Work out the finished part from the listing and answer in its coordinate system (mm). A direction names the side the tool comes from. Round coordinates to 2 decimals unless told otherwise and drop trailing zeros. Order: outer loops, then holes, each group sorted by start corner. A loop starts at its lowest first (then second) coordinate and runs counter-clockwise, first axis right, second up. Notation, with made-up numbers: (45, 32.5) - (96, 32.5) arc R24 ccw to (96, 54.5) - close; hole circle Ø3 at (79.5, 18.25). An arc over 180 degrees is marked (long way). Answer in a Markdown table with one row per item.
from build123d import *

# Parameters (mm, degrees)
SKETCH1_R           = 4.1
SKETCH1_R_2         = 4
SKETCH1_R_3         = 2.6
BOSS_EXTRUDE1_DEPTH = 10
CUT_EXTRUDE1_START  = -4
CUT_EXTRUDE1_DEPTH  = 4
FILLET1_R           = 2
BOSS_EXTRUDE2_START = -20
SKETCH3_R           = 4
BOSS_EXTRUDE2_DEPTH = 20
FILLET2_R           = 1
CUT_EXTRUDE2_REACH  = 75.469


with BuildPart() as part:
    # Sketch1 → Boss-Extrude1 (new body)
    with BuildSketch(Plane(origin=(0, 0, 0), x_dir=(1, 0, 0), z_dir=(0, 1, 0))):
        with BuildLine():
            Line((11.273947383, 72.313413723), (4.792068361, 72.313413723))
            Line((4.792068361, 72.313413723), (-53.726052617, 72.313413723))
            ThreePointArc((-53.726052617, 72.313413723), (-57.261586523, 70.848947629), (-58.726052617, 67.313413723))
            Line((-58.726052617, 67.313413723), (-58.726052617, 34.313413723))
            ThreePointArc((-58.726052617, 34.313413723), (-57.261586523, 30.777879817), (-53.726052617, 29.313413723))
            Line((-53.726052617, 29.313413723), (-5.726052617, 29.313413723))
            ThreePointArc((-5.726052617, 29.313413723), (1.345015195, 26.384481534), (4.273947383, 19.313413723))
            Line((4.273947383, 19.313413723), (4.273947383, 17.313413723))
            ThreePointArc((4.273947383, 17.313413723), (5.738413477, 13.777879817), (9.273947383, 12.313413723))
            Line((9.273947383, 12.313413723), (36.273947383, 12.313413723))
            ThreePointArc((36.273947383, 12.313413723), (39.809481289, 13.777879817), (41.273947383, 17.313413723))
            Line((41.273947383, 17.313413723), (41.273947383, 42.313413723))
            ThreePointArc((41.273947383, 42.313413723), (32.487150819, 63.526617158), (11.273947383, 72.313413723))
        make_face()
        with Locations(Location((33.273947383, 20.313413723, 0), (0, 0, 270))):
            Circle(SKETCH1_R, mode=Mode.SUBTRACT)
        with Locations(Location((12.273947383, 20.313413723, 0), (0, 0, 270))):
            Circle(SKETCH1_R_2, mode=Mode.SUBTRACT)
        with Locations(Location((-50.726052617, 64.313413723, 0), (0, 0, 270))):
            Circle(SKETCH1_R_3, mode=Mode.SUBTRACT)
        with Locations(Location((-50.726052617, 37.313413723, 0), (0, 0, 270))):
            Circle(SKETCH1_R_3, mode=Mode.SUBTRACT)
        with BuildLine():
            Line((34.171420048, 34.313413723), (26.134777641, 34.313413723))
            ThreePointArc((26.134777641, 34.313413723), (25.561526201, 34.49403421), (25.19535667, 34.97064815))
            Line((25.19535667, 34.97064815), (14.615821544, 63.966084002))
            ThreePointArc((14.615821544, 63.966084002), (14.998488248, 65.980552022), (16.952543045, 66.601989919))
            ThreePointArc((16.952543045, 66.601989919), (32.892900514, 54.755368869), (35.127730175, 35.021059585))
            ThreePointArc((35.127730175, 35.021059585), (34.766250218, 34.509562325), (34.171420048, 34.313413723))
        make_face(mode=Mode.SUBTRACT)
        with BuildLine():
            Line((-42.557674575, 35.313413723), (-42.557674575, 60.452375226))
            ThreePointArc((-42.557674575, 60.452375226), (-41.891342574, 61.395065879), (-40.780343242, 61.081466633))
            Line((-40.780343242, 61.081466633), (-20.435473581, 35.94250513))
            ThreePointArc((-20.435473581, 35.94250513), (-20.310283056, 34.882769674), (-21.212804914, 34.313413723))
            Line((-21.212804914, 34.313413723), (-41.557674575, 34.313413723))
            ThreePointArc((-41.557674575, 34.313413723), (-42.264781356, 34.606306941), (-42.557674575, 35.313413723))
        make_face(mode=Mode.SUBTRACT)
        with BuildLine():
            Line((-37.245793747, 67.251595954), (5.443945576, 67.251595954))
            ThreePointArc((5.443945576, 67.251595954), (6.346467434, 66.682240002), (6.221276909, 65.622504547))
            Line((6.221276909, 65.622504547), (-15.123592752, 39.247901728))
            ThreePointArc((-15.123592752, 39.247901728), (-15.900924085, 38.876993135), (-16.678255419, 39.247901728))
            Line((-16.678255419, 39.247901728), (-38.02312508, 65.622504547))
            ThreePointArc((-38.02312508, 65.622504547), (-38.148315604, 66.682240002), (-37.245793747, 67.251595954))
        make_face(mode=Mode.SUBTRACT)
        with BuildLine():
            Line((19.622800135, 35.656179295), (10.526467022, 60.58658882))
            ThreePointArc((10.526467022, 60.58658882), (9.751557094, 61.230198488), (8.809714717, 60.872914654))
            Line((8.809714717, 60.872914654), (-11.36637459, 35.94250513))
            ThreePointArc((-11.36637459, 35.94250513), (-11.491565114, 34.882769674), (-10.589043257, 34.313413723))
            Line((-10.589043257, 34.313413723), (18.683379163, 34.313413723))
            ThreePointArc((18.683379163, 34.313413723), (19.502758676, 34.740162282), (19.622800135, 35.656179295))
        make_face(mode=Mode.SUBTRACT)
    extrude(amount=BOSS_EXTRUDE1_DEPTH)

    # Sketch2 → Cut-Extrude1 (cut)
    with BuildSketch(Plane(origin=(0, 10, 0), x_dir=(1, 0, 0), z_dir=(0, 1, 0)).offset(CUT_EXTRUDE1_START)):
        with BuildLine():
            Line((33.273947383, 27.813413723), (41.273947383, 27.813413723))
            Line((41.273947383, 27.813413723), (41.273947383, 17.313413723))
            ThreePointArc((41.273947383, 17.313413723), (39.809481289, 13.777879817), (36.273947383, 12.313413723))
            Line((36.273947383, 12.313413723), (25.773947383, 12.313413723))
            Line((25.773947383, 12.313413723), (25.773947383, 20.313413723))
            ThreePointArc((25.773947383, 20.313413723), (27.970646524, 25.616714582), (33.273947383, 27.813413723))
        make_face()
    extrude(amount=CUT_EXTRUDE1_DEPTH, mode=Mode.SUBTRACT)

    # Fillet1
    fillet1_edges = [part.edges().sort_by_distance(p)[0] for p in [
        (41.273947383, 8, -27.813413723),
        (25.773947383, 8, -12.313413723),
    ]]
    fillet(fillet1_edges, radius=FILLET1_R)

    # Sketch3 → Boss-Extrude2 (add)
    with BuildSketch(Plane(origin=(0, 10, 0), x_dir=(1, 0, 0), z_dir=(0, 1, 0)).offset(BOSS_EXTRUDE2_START)):
        with Locations(Location((12.273947383, 20.313413723, 0), (0, 0, 270))):
            Circle(SKETCH3_R)
    extrude(amount=BOSS_EXTRUDE2_DEPTH)

    # Fillet2
    fillet2_edges = [part.edges().sort_by_distance(p)[0] for p in [
        (12.273947383, -10, -24.313413723),
        (12.273947383, 0, -24.313413723),
    ]]
    fillet(fillet2_edges, radius=FILLET2_R)

    # Cut-Extrude2: up to this face of the body (flat: up to its plane)
    cut_extrude2_end = Plane(part.part.faces().sort_by_distance((-21.226052617, 5, -72.313413723))[0])
    # Sketch4 → Cut-Extrude2 (cut, up to the picked face)
    with BuildSketch(Plane.XY.offset(-29.313413723), mode=Mode.PRIVATE) as cut_extrude2_sk1:
        Polygon((-5.726052617, 10), (-41.726052617, 5), (-62.366339881, 5), (-62.366339881, 10), align=None)
    cut_extrude2_tool1 = split(extrude(cut_extrude2_sk1.sketch, amount=-CUT_EXTRUDE2_REACH, mode=Mode.PRIVATE), bisect_by=cut_extrude2_end, keep=Keep.BOTH, mode=Mode.PRIVATE)
    add(cut_extrude2_tool1.solids().sort_by(Axis((-41.648691, 7.888196, -29.313414), (0, 0, -1)))[0], mode=Mode.SUBTRACT)


solid = part.part
1) Which of the six approach directions +Z, -Z, +X, -X, +Y, -Y give full straight-line access (tool end or side, diameter ignored) to faces 5 (the face through (4.274, 5, -18)), 6 (the face through (37, 6, -17)), 7 (the face through (14.98, -5.06, -23.26)), 8 (the face through (-41.91, 2.53, -61.39))?
Filled in:
| item | result |
|---|---|
| face 5 | +Z, -X, +Y, -Y |
| face 6 | +Z, +X, +Y |
| face 7 | -Y |
| face 8 | +Y, -Y |
2) Find section B-B, the plane z = -53. Give the vertices of the cut face in (x, y).
Filled in:
| item | result |
|---|---|
| outline | (-58.73, 0) - (-42.56, 0) - (-42.56, 5) - (-58.73, 5) - close; (-34.24, 0) - (-27.81, 0) - (-27.81, 6.93) - (-34.24, 6.04) - close; (-3.99, 0) - (2.44, 0) - (2.44, 10) - (-3.99, 10) - close; (13.29, 0) - (18.62, 0) - (18.62, 10) - (13.29, 10) - close; (33.81, 0) - (39.31, 0) - (39.31, 10) - (33.81, 10) - close |
3) Each of these flat-tipped pins is pushed along its axis until it touches: pin 1 (10 mm diameter, centred on y = 3, z = -62.5, fed in from +X); pin 2 (4 mm diameter, centred on y = 3, z = -47.5, fed in from +X); pin 3 (2 mm diameter, centred on x = 37.5, y = 9, fed in from +Z); pin 4 (3 mm diameter, centred on y = 4, z = -34, fed in from -X). Where does it stop, or does it pass through?
Filled in:
| item | result |
|---|---|
| pin 1 | stops at x = 37.15 |
| pin 2 | stops at x = 41.1 |
| pin 3 | stops at z = -27.81 |
| pin 4 | stops at x = -58.73 |
4) Find section A-A, the plane x = -23.5. Give the vertices of the cut face in (y, z), then the cut area to 3 significant figures.
Filled in:
| item | result |
|---|---|
| outline | (0, -72.31) - (7.53, -72.31) - (7.53, -67.25) - (0, -67.25) - close; (0, -47.68) - (7.53, -47.68) - (7.53, -39.73) - (0, -39.73) - close; (0, -34.31) - (7.53, -34.31) - (7.53, -29.31) - (0, -29.31) - close |
| area | 136 mm^2 |
5) Find section C-C, the plane x = -35. Give the vertices of the cut face in (y, z), then the cut area to 3 significant figures.
Filled in:
| item | result |
|---|---|
| outline | (0, -72.31) - (5.93, -72.31) - (5.93, -67.25) - (0, -67.25) - close; (0, -61.89) - (5.93, -61.89) - (5.93, -53.94) - (0, -53.94) - close; (0, -34.31) - (5.93, -34.31) - (5.93, -29.31) - (0, -29.31) - close |
| area | 107 mm^2 |
6) Find the intervals of material crossed by probe 1 along X at (y, z) = (5.5, -20); probe 2 along Z at (x, y) = (9.5, 2.75); probe 3 along Z at (x, y) = (33, 1.75), in increasing order. Write a range as from..to.
Filled in:
| item | result |
|---|---|
| probe 1 | x = 4.25..29.19, 37.36..41.27 |
| probe 2 | z = -72.31..-61.24, -34.31..-12.31 |
| probe 3 | z = -63..-54.57, -34.31..-24.4, -16.22..-12.31 |
7) The mould has two halves that part along Z. Classify faces 1 (the face through (25.17, 8.03, -12.88)), 2 (the face through (32.75, 4.93, -55)), 3 (the face through (-58.726, 2, -51)), 4 (the face through (-16, 4, -67.252)): released by +Z, released by -Z, zero draft, split by the parting line, or undercut.
Filled in:
| item | result |
|---|---|
| face 1 | released by +Z |
| face 2 | undercut |
| face 3 | zero draft |
| face 4 | undercut |
8) Find section D-D, the plane y = -2. Give the vertices of the cut face in (x, z).
Filled in:
| item | result |
|---|---|
| outline | circle Ø8 at (12.27, -20.31) |
